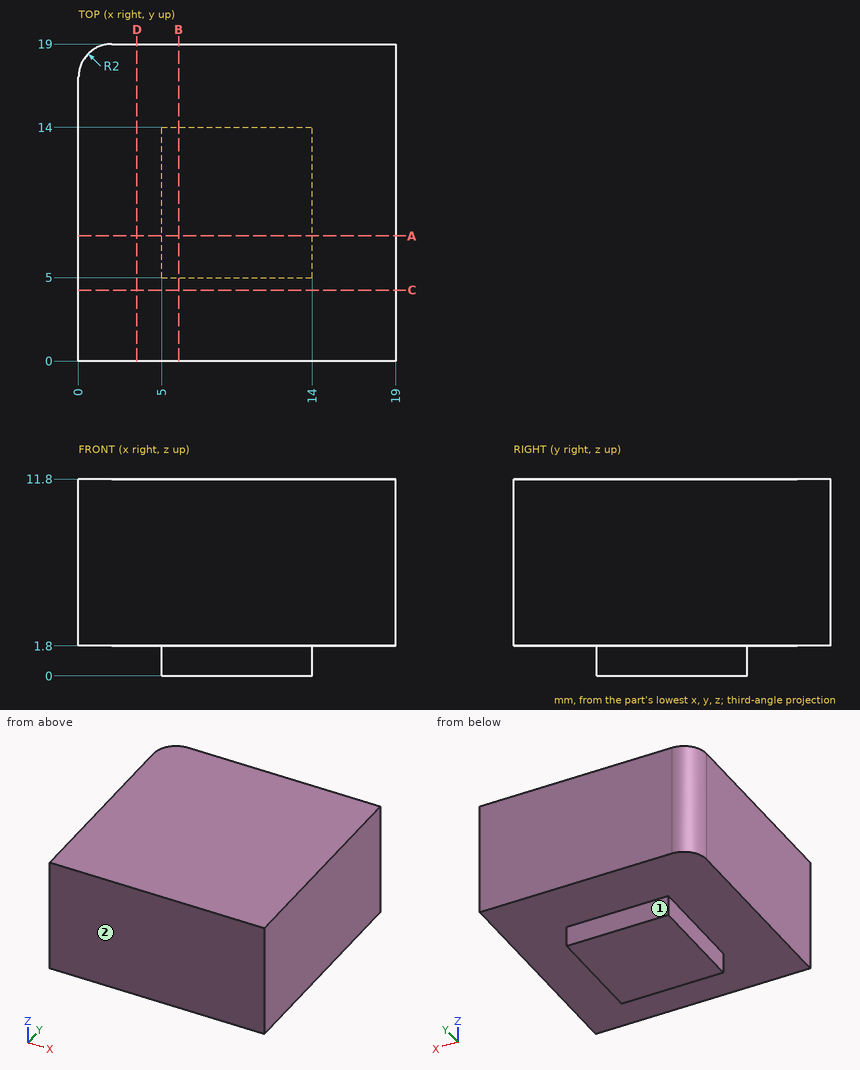
Design review of the part shown in the three views and the two pictorial views. Dimensions are in mm from the part's minimum x, y and z. A direction names the side the tool comes from. Round coordinates to 2 decimals unless told otherwise and drop trailing zeros. Loops run counter-clockwise (first coordinate to the right, second up) from the corner with the lowest first, then second, coordinate; pieces in that order, holes last. Notation, with made-up numbers: (39.5, 73.5) - (90.5, 73.5) arc R11 cw to (90.5, 81.5) - close; hole circle Ø10 at (29.5, 56). An arc over 180 degrees is marked (long way). Use CSV: the item, a comma, the result in double quotes.
(1) Take a section at C-C, the plane y = 4.25. Give the boundary of the cut face in (x, z).
Working result:
outline,"(0, 1.8) - (19, 1.8) - (19, 11.8) - (0, 11.8) - close"
(2) Take a section at A-A, the plane y = 7.5. Give the boundary of the cut face in (x, z), plus the area to 3 significant figures.
Working result:
outline,"(0, 1.8) - (5, 1.8) - (5, 0) - (14, 0) - (14, 1.8) - (19, 1.8) - (19, 11.8) - (0, 11.8) - close"
area,"206 mm^2"
(3) Clearance check with flat-ended pins moving along their axes: P1, Ø1.5, axis at x = 12.5, y = 8, coming from the -Z side; P2, Ø0.9, axis at y = 11, z = 0.5, coming from the +X side; P3, Ø2, axis at x = 8, z = 0.5, coming from the +Y side; P4, Ø0.5, axis at x = 8.5, z = 1.5, coming from the -Y side. State where each tip first meets the part, or that it passes through.
Working result:
P1,"stops at z = 0"
P2,"stops at x = 14"
P3,"stops at y = 14"
P4,"stops at y = 5"
(4) For line 1 (Z direction, x = 9.25, y = 1.75); line 2 (X direction, y = 17.75, z = 10.25), list the stretches that pass through material, from the lowest coordinate up.
Working result:
line 1,"z = 1.8 to 11.8"
line 2,"x = 0.15 to 19"
(5) Machinability: for the marked faces 1 and 2, which of the approach directions +Z, -Z, +X, -X, +Y, -Y give a long, thin tool a straight path to every point of the face, cutting with its end or side? Answer none if there is none.
Working result:
face 1,"-Z, +X, -X, +Y"
face 2,"+Z, -Z, +X, -X, -Y"
